Here's how the part is built. I have some questions about the finished solid (model axes, mm). Face numbers are marked on the shaded views. Coordinates: 2 decimals unless noted, no trailing zeros. Loops run counter-clockwise (first coordinate to the right, second up) from the corner with the lowest first, then second, coordinate; pieces in that order, holes last. Notation, with made-up numbers: M 5,-17 L 34,-17 A14 cw 34,3 Z; hole C -20,41.25 d11. An arc over 180 degrees is marked long. Use CSV: the item, a comma, the result in double quotes. Start each with the question number.
Q1. If we section it at D-D (x = 3): Please give me the cut outline in (y, z), and give its area (3 significant figures).
Q2. If we section it at B-B (y = -1.75): Please give me the cut outline in (x, z).
Q3. If we mould it in two halves opening along X, with no side actions, what happens to the marked faces 1, 2 and 3? For each: +X half, -X half, draft (parallel to the pull), parting line (faces both ways), or undercut.
Q4. If we section it at A-A (z = 0): Please give me the cut outline in (x, y).
Q5. If we section it at C-C (x = -3): Please give me the cut outline in (y, z).
Q6. For pin 1 Ø3 at (x, y) = (17.5, 0) entering from -Z; pin 2 Ø0.6 at (x, y) = (47.5, 3.5) entering from +Z; pin 3 Ø0.6 at (y, z) = (-2, -2.5) entering from -X, each with a flat end and sliding along its axis, tell me the tip position at first contact or that it passes through.
Q7. Please list where these lines run through material, in increasing order: probe 1 along X at (y, z) = (1.75, 3.25); probe 2 along Z at (x, y) = (18, 0.25); probe 3 along Y at (x, z) = (4.5, 0). Write a range as [from, to].
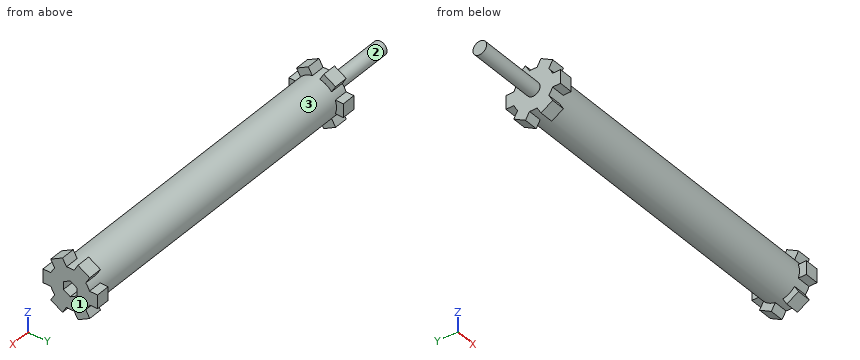
from build123d import *

# Parameters (mm, degrees)
ESBO_O1_R                 = 3
RESSALTO_EXTRUS_O1_DEPTH  = 48
ESBO_O2_W                 = 4
ESBO_O2_H                 = 2
RESSALTO_EXTRUS_O2_DEPTH  = 4
ESBO_O4_R                 = 4.471241999
CORTE_EXTRUS_O2_DEPTH     = 2
PADR_OCIRCULAR1_COUNT     = 6
ESBO_O7_R                 = 7.725132362
CORTE_EXTRUS_O3_DEPTH     = 2
ESPELHAR5_COPY_1_SKETCH_W = 4
ESPELHAR5_COPY_1_SKETCH_H = 2
ESPELHAR5_COPY_1_DEPTH    = 4
ESPELHAR5_COPY_2_SKETCH_W = 4
ESPELHAR5_COPY_2_SKETCH_H = 2
ESPELHAR5_COPY_2_DEPTH    = 4
ESPELHAR5_COPY_3_SKETCH_W = 4
ESPELHAR5_COPY_3_SKETCH_H = 2
ESPELHAR5_COPY_3_DEPTH    = 4
ESPELHAR5_COPY_4_SKETCH_W = 4
ESPELHAR5_COPY_4_SKETCH_H = 2
ESPELHAR5_COPY_4_DEPTH    = 4
ESPELHAR5_COPY_5_SKETCH_W = 4
ESPELHAR5_COPY_5_SKETCH_H = 2
ESPELHAR5_COPY_5_DEPTH    = 4
ESBO_O10_R                = 7.180900458
CORTE_EXTRUS_O5_DEPTH     = 2
ESBO_O11_R                = 1
RESSALTO_EXTRUS_O3_DEPTH  = 10
CORTE_EXTRUS_O6_DEPTH     = 3


with BuildPart() as part:
    # Esboço1 → Ressalto-extrusão1 (new body)
    with BuildSketch(Plane(origin=(0, 0, 0), x_dir=(0, 0, -1), z_dir=(1, 0, 0))):
        Circle(ESBO_O1_R)
    ressalto_extrus_o1 = extrude(amount=RESSALTO_EXTRUS_O1_DEPTH)

    # Esboço2 → Ressalto-extrusão2 (add, symmetric)
    with BuildSketch(Plane(origin=(0, 0, 0), x_dir=(1, 0, 0), z_dir=(0, 1, 0))):
        Rectangle(ESBO_O2_W, ESBO_O2_H)
    ressalto_extrus_o2 = extrude(amount=RESSALTO_EXTRUS_O2_DEPTH, both=True)

    # Esboço4 → Corte-extrusão2 (cut)
    with BuildSketch(Plane.ZY.offset(2)):
        Circle(ESBO_O4_R)
    extrude(amount=-CORTE_EXTRUS_O2_DEPTH, mode=Mode.SUBTRACT)

    # PadrãoCircular1: Ressalto-extrusão2 ×6 about axis
    padr_ocircular1_axis = Axis((0, 0, 0), (1, 0, 0))
    for i in range(1, PADR_OCIRCULAR1_COUNT):
        add(ressalto_extrus_o2.rotate(padr_ocircular1_axis, i * 360 / PADR_OCIRCULAR1_COUNT))

    # Esboço7 → Corte-extrusão3 (cut)
    with BuildSketch(Plane.ZY.offset(2)):
        Circle(ESBO_O7_R)
    extrude(amount=-CORTE_EXTRUS_O3_DEPTH, mode=Mode.SUBTRACT)

    # Espelhar5: Ressalto-extrusão1, Ressalto-extrusão2 across plane
    add(ressalto_extrus_o1.mirror(Plane(origin=(24, 0, 0), x_dir=(0, 0, 1), z_dir=(1, 0, 0))))
    add(ressalto_extrus_o2.mirror(Plane(origin=(24, 0, 0), x_dir=(0, 0, 1), z_dir=(1, 0, 0))))

    # Espelhar5 copy 1 sketch → Espelhar5 copy 1 (add, symmetric)
    with BuildSketch(Plane(origin=(48, 0, 0), x_dir=(-1, 0, 0), z_dir=(0, 0.5, 0.866025404))):
        Rectangle(ESPELHAR5_COPY_1_SKETCH_W, ESPELHAR5_COPY_1_SKETCH_H)
    extrude(amount=ESPELHAR5_COPY_1_DEPTH, both=True)

    # Espelhar5 copy 2 sketch → Espelhar5 copy 2 (add, symmetric)
    with BuildSketch(Plane(origin=(48, 0, 0), x_dir=(-1, 0, 0), z_dir=(0, -0.5, 0.866025404))):
        Rectangle(ESPELHAR5_COPY_2_SKETCH_W, ESPELHAR5_COPY_2_SKETCH_H)
    extrude(amount=ESPELHAR5_COPY_2_DEPTH, both=True)

    # Espelhar5 copy 3 sketch → Espelhar5 copy 3 (add, symmetric)
    with BuildSketch(Plane(origin=(48, 0, 0), x_dir=(-1, 0, 0), z_dir=(0, -1, 0))):
        Rectangle(ESPELHAR5_COPY_3_SKETCH_W, ESPELHAR5_COPY_3_SKETCH_H)
    extrude(amount=ESPELHAR5_COPY_3_DEPTH, both=True)

    # Espelhar5 copy 4 sketch → Espelhar5 copy 4 (add, symmetric)
    with BuildSketch(Plane(origin=(48, 0, 0), x_dir=(-1, 0, 0), z_dir=(0, -0.5, -0.866025404))):
        Rectangle(ESPELHAR5_COPY_4_SKETCH_W, ESPELHAR5_COPY_4_SKETCH_H)
    extrude(amount=ESPELHAR5_COPY_4_DEPTH, both=True)

    # Espelhar5 copy 5 sketch → Espelhar5 copy 5 (add, symmetric)
    with BuildSketch(Plane(origin=(48, 0, 0), x_dir=(-1, 0, 0), z_dir=(0, 0.5, -0.866025404))):
        Rectangle(ESPELHAR5_COPY_5_SKETCH_W, ESPELHAR5_COPY_5_SKETCH_H)
    extrude(amount=ESPELHAR5_COPY_5_DEPTH, both=True)

    # Esboço10 → Corte-extrusão5 (cut)
    with BuildSketch(Plane(origin=(50, 0, 0), x_dir=(0, 0, -1), z_dir=(1, 0, 0))):
        Circle(ESBO_O10_R)
    extrude(amount=-CORTE_EXTRUS_O5_DEPTH, mode=Mode.SUBTRACT)

    # Esboço11 → Ressalto-extrusão3 (add)
    with BuildSketch(Plane.ZY):
        Circle(ESBO_O11_R)
    extrude(amount=RESSALTO_EXTRUS_O3_DEPTH)

    # Esboço12 → Corte-extrusão6 (cut)
    with BuildSketch(Plane(origin=(48, 0, 0), x_dir=(0, 0, -1), z_dir=(1, 0, 0))):
        Polygon((-0.577350269, 1), (-1.154700538, 0), (-0.577350269, -1), (0.577350269, -1), (1.154700538, 0), (0.577350269, 1), align=None)
    extrude(amount=-CORTE_EXTRUS_O6_DEPTH, mode=Mode.SUBTRACT)


solid = part.part
Results below:
1,outline,"C 0,0 d6"
1,area,"28.3 mm^2"
2,outline,"M 0,-3.61 L 2,-3.61 L 2,-2.44 L 46,-2.44 L 46,-3.61 L 48,-3.61 L 48,3.61 L 46,3.61 L 46,2.44 L 2,2.44 L 2,3.61 L 0,3.61 Z"
3,face 1,"+X half"
3,face 2,"draft"
3,face 3,"undercut"
4,outline,"M -10,-1 L 0,-1 L 0,-4 L 2,-4 L 2,-3 L 46,-3 L 46,-4 L 48,-4 L 48,-1 L 45,-1 L 45,1 L 48,1 L 48,4 L 46,4 L 46,3 L 2,3 L 2,4 L 0,4 L 0,1 L -10,1 Z"
5,outline,"C 0,0 d2"
6,pin 1,"z = -3"
6,pin 2,"z = 1"
6,pin 3,"x = 0"
7,probe 1,"[0, 2], [46, 48]"
7,probe 2,"[-2.99, 2.99]"
7,probe 3,"[-3, 3]"
